Part model, mm, in its own coordinate system. Coordinates: 2 decimals unless noted, no trailing zeros. Loops run counter-clockwise (first coordinate to the right, second up) from the corner with the lowest first, then second, coordinate; pieces in that order, holes last. Notation, with made-up numbers: (49.25, 48) - (90.25, 48) arc R12 cw to (90.25, 60) - close; hole circle Ø2 at (0.5, 72). An arc over 180 degrees is marked (long way). Use a Markdown table: item, result. Add a question column.
1) Band-saw the part on B-B (y = 11). Give the cut face in (x, z), plus the area to 3 significant figures.
2) Probe probe 1 along Y at (x, z) = (1283, 4.25). List the from-to ranges inside material, lowest first. Write a range as [from, to].
3) Band-saw the part on A-A (z = 2.5). Give the cut face in (x, y), plus the area to 3 significant figures.
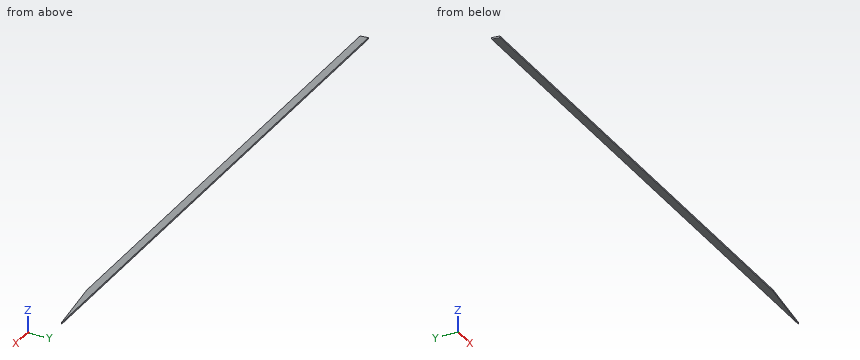
from build123d import *

# Parameters (mm, degrees)
F0_W     = 2971.96
F0_H     = 40
F1_DEPTH = 8
F3_DEPTH = 100
F5_DEPTH = 25
F7_DEPTH = 25


with BuildPart() as f1:
    # F0 (on Top) → F1 (new body)
    with BuildSketch(Plane.XY):
        Rectangle(F0_W, F0_H)
    extrude(amount=F1_DEPTH)

    # F2 (on face) → F3 (cut)
    with BuildSketch(Plane.XY.offset(8)):
        Polygon((1485.98, -20), (1485.98, 20), (1159.31062, -20), align=None)
    extrude(amount=-F3_DEPTH, mode=Mode.SUBTRACT)

    # F4 (on face) → F5 (cut)
    with BuildSketch(Plane.XY.offset(8)):
        Polygon((1475.98, 18.77552), (1485.98, 20), (1475.98, 20), align=None)
    extrude(amount=-F5_DEPTH, mode=Mode.SUBTRACT)

    # F6 (on face) → F7 (cut)
    with BuildSketch(Plane.XY.offset(8)):
        Polygon((-1481.082081, -20), (-1485.98, 20), (-1485.98, -20), align=None)
    extrude(amount=-F7_DEPTH, mode=Mode.SUBTRACT)


solid = f1.part
Answer block:
| question | item | result |
|---|---|---|
| 1 | outline | (-1484.88, 0) - (1412.48, 0) - (1412.48, 8) - (-1484.88, 8) - close |
| 1 | area | 23,200 mm2 |
| 2 | probe 1 | [-4.85, 20] |
| 3 | outline | (-1485.98, 20) - (-1481.08, -20) - (1159.31, -20) - (1475.98, 18.78) - (1475.98, 20) - close |
| 3 | area | 112,000 mm2 |
